from build123d import *

# Parameters (mm, degrees)
F1_DEPTH  = 16
F2_W      = 64
F2_H      = 16
F3_DEPTH  = 48
F4_R      = 32
F5_W      = 42
F5_H      = 40
F6_DEPTH  = 28
F8_DEPTH  = 50
F9_W      = 12
F9_H      = 40
F10_DEPTH = 28
F12_W     = 12
F12_H     = 48.826222
F13_DEPTH = 25


with BuildPart() as f1:
    # F0 (on Top) → F1 (new body)
    with BuildSketch(Plane.XY):
        with BuildLine():
            Line((-19.074771, -39.273684), (44.925229, -39.273684))
            Line((44.925229, -39.273684), (44.925229, 56.726316))
            Line((44.925229, 56.726316), (28.229578, 56.726316))
            Line((28.229578, 56.726316), (28.229578, 36.726316))
            ThreePointArc((28.229578, 36.726316), (20.229578, 28.726316), (12.229578, 36.726316))
            Line((12.229578, 36.726316), (12.229578, 56.726316))
            Line((12.229578, 56.726316), (-19.074771, 56.726316))
            Line((-19.074771, 56.726316), (-19.074771, -39.273684))
        make_face()
    extrude(amount=F1_DEPTH)

    # F2 (on face) → F3 (join)
    with BuildSketch(Plane.XY.offset(16)):
        with Locations((12.925229, -31.273684)):
            Rectangle(F2_W, F2_H)
    extrude(amount=F3_DEPTH)

    # F4
    f4_edges = [f1.edges().sort_by_distance(p)[0] for p in [
        (44.925229, -31.273684, 64),
    ]]
    fillet(f4_edges, radius=F4_R)

    # F5 (on face) → F6 (join)
    with BuildSketch(Plane.XY.offset(16)):
        with Locations((1.925229, -3.273684)):
            Rectangle(F5_W, F5_H)
    extrude(amount=F6_DEPTH)

    # F7 (on face) → F8 (cut)
    with BuildSketch(Plane.YZ.offset(22.925229)):
        with BuildLine():
            Line((8.726316, 44), (-15.273684, 44))
            ThreePointArc((-15.273684, 44), (-3.273684, 32), (8.726316, 44))
        make_face()
    extrude(amount=-F8_DEPTH, mode=Mode.SUBTRACT)

    # F9 (on face) → F10 (join)
    with BuildSketch(Plane.XY.offset(16)):
        with Locations((-13.074771, 36.726316)):
            Rectangle(F9_W, F9_H)
    extrude(amount=F10_DEPTH)

    # F12 (on face) → F13 (cut)
    with BuildSketch(Plane(origin=(0, 26.171742, 37.388202), x_dir=(1, 0, 0), z_dir=(0, 0.573462, 0.819232))):
        with Locations((-13.074771, 12.8835)):
            Rectangle(F12_W, F12_H)
    extrude(amount=F13_DEPTH, mode=Mode.SUBTRACT)


solid = f1.part
Verification items for the finished model (mm, model axes). A direction names the side the tool comes from. Coordinates: 2 decimals unless noted, no trailing zeros. Write each loop counter-clockwise with the first axis right and the second up, starting at its lowest first coordinate (ties: lowest second). Pieces come first, ordered by that corner, then holes. Notation, with made-up numbers: M 28,-13.75 L 48,-13.75 A23 ccw 48,20.25 Z; hole C 60.25,35 d2. An arc over 180 degrees is marked long. Use a Markdown table: item, result.
Q1. Go/stop test with flat-tipped pins: P1, Ø22.5, axis at x = 9.5, z = 25.5, coming from the +Y side; P2, Ø4, axis at x = 0.5, z = 42.5, coming from the +Y side; P3, Ø22.5, axis at y = -0.5, z = 28.5, coming from the +X side; P4, Ø2.5, axis at x = 12, y = 13, coming from the +Z side. Record where each tip stops, or that it passes through.
Reply:
| item | result |
|---|---|
| P1 | stops at y = 56.73 |
| P2 | stops at y = 16.73 |
| P3 | stops at x = 22.93 |
| P4 | stops at z = 44 |
Q2. Draft check along Y on faces 6 (the face through (2, -19, 44)), 7 (the face through (20.41, 28.73, 7.89)), 8 (the face through (2.219, -3.538, 32.003)). Enter one of: +Y half, -Y half, draft (parallel to the pull), parting line (faces both ways), or undercut.
Reply:
| item | result |
|---|---|
| face 6 | draft |
| face 7 | +Y half |
| face 8 | undercut |
Q3. Thickness scan on line 1 (Y direction, x = 24, z = 61.5); line 2 (X direction, y = 31, z = 13); line 3 (X direction, y = 33.5, z = 23). Record the ranges inside material, lowest first.
Reply:
| item | result |
|---|---|
| line 1 | y = -39.27 to -23.27 |
| line 2 | x = -19.07 to 14.64, 25.82 to 44.93 |
| line 3 | x = -19.07 to -7.07 |
Q4. Sectioned sample at C-C, the plane z = 11.5. Record the boundary of the cut face in (x, y).
Reply:
| item | result |
|---|---|
| outline | M -19.07,-39.27 L 44.93,-39.27 L 44.93,56.73 L 28.23,56.73 L 28.23,36.73 A8 cw 12.23,36.73 L 12.23,56.73 L -19.07,56.73 Z |
Q5. Sectioned sample at A-A, the plane y = 32. Record the boundary of the cut face in (x, z), plus the area to 3 significant figures.
Reply:
| item | result |
|---|---|
| outline | M -19.07,0 L 13.77,0 L 13.77,16 L -7.07,16 L -7.07,33.31 L -19.07,33.31 Z; M 26.68,0 L 44.93,0 L 44.93,16 L 26.68,16 Z |
| area | 1,030 mm² |
Q6. Set-up check for faces 1 (the face through (-7.075, 32, 27)), 2 (the face through (12.23, 47, 8)), 3 (the face through (12, 9, 0)), 4 (the face through (44.925, -3, 12)), 5 (the face through (2, 13, 44)): record each of +Z, -Z, +X, -X, +Y, -Y from which the full face is reachable in a straight line by a thin tool's end or side.
Reply:
| item | result |
|---|---|
| face 1 | +Z, +X, +Y |
| face 2 | +Z, -Z, +Y |
| face 3 | -Z, +X, -X, +Y, -Y |
| face 4 | +Z, -Z, +X, +Y, -Y |
| face 5 | +Z, +X, -X, +Y |
Q7. Sectioned sample at D-D, the plane y = 12.5. Record the boundary of the cut face in (x, z).
Reply:
| item | result |
|---|---|
| outline | M -19.07,0 L 44.93,0 L 44.93,16 L 22.93,16 L 22.93,44 L -19.07,44 Z |
